Here's how the part is built. I have some questions about the finished solid (model axes, mm). A direction names the side the tool comes from. Coordinates: 2 decimals unless noted, no trailing zeros. Write each loop counter-clockwise with the first axis right and the second up, starting at its lowest first coordinate (ties: lowest second). Pieces come first, ordered by that corner, then holes.
Item 1: I want a section at B-B (z = -5). Please give me the cut outline in (x, y) (3 decimals), and give its area (3 significant figures).
Item 2: I want a section at C-C (y = 10.25). Please give me the cut outline in (x, z) (3 decimals).
Item 3: Please list where these lines run through material, in increasing order: line 1 (Y direction, x = 25, z = 0.5); line 2 (X direction, y = 3, z = 0.75) (3 decimals); line 3 (X direction, y = 4.5, z = -3) (3 decimals).
Item 4: If we mould it in two halves opening along X, with no side actions, what happens to faces 4 (the face through (62.103, 10, 3)), 5 (the face through (61.595, 10, 3)), 6 (the face through (22.71, 21.45, 0.09))? For each: pulls with the +X half, pulls with the -X half, needs draft (parallel to the pull), parting line crosses it, or undercut.
Item 5: I want a section at A-A (x = 52.5). Please give me the cut outline in (y, z), and give its area (3 significant figures).
Item 6: I want a section at D-D (z = 2.75). Please give me the cut outline in (x, y) (3 decimals), and give its area (3 significant figures).
Item 7: For faces 1 (the face through (1, 0.508, 0)), 2 (the face through (61.213, 20.72, 0.088)), 3 (the face through (1, 0, 0)), which set-ups out of +Z, -Z, +X, -X, +Y, -Y let a thin tool reach every point of the face, with its end or its side?
Item 8: I'm going to push flat-ended pins straight in: P1, Ø4, axis at x = 45.5, z = -1.5, coming from the +Y side; P2, Ø4, axis at x = 45, z = 0, coming from the -Y side; P3, Ø4, axis at y = 12.5, z = -4, coming from the -X side; P4, Ø0.6, axis at x = 62, z = -1, coming from the +Y side. Where does each tip first touch, or does it pass through?
from build123d import *

# Parameters (mm, degrees)
EXTRUDE_THIN1_DEPTH = 6.3119
CUT_EXTRUDE1_REACH  = 68.051
SKETCH2_W           = 4.318
SKETCH2_H           = 11.049
CUT_EXTRUDE2_REACH  = 68.051
SKETCH3_R           = 1.524
SKETCH3_R_2         = 3.4925


with BuildPart() as part:
    # Sketch1 → Extrude-Thin1 (new, symmetric)
    with BuildSketch(Plane.XY):
        with BuildLine():
            Line((0, 0), (1.784287341, 0))
            ThreePointArc((1.784287341, 0), (2.479784243, 0.141672386), (3.064445706, 0.54411242))
            Line((3.064445706, 0.54411242), (22.485395925, 20.693348272))
            ThreePointArc((22.485395925, 20.693348272), (22.903011255, 20.980805438), (23.399794757, 21.082))
            Line((23.399794757, 21.082), (60.325, 21.082))
            ThreePointArc((60.325, 21.082), (61.223025612, 20.710025612), (61.595, 19.812))
            Line((61.595, 19.812), (61.595, 0))
            Line((61.595, 0), (62.103, 0))
            Line((62.103, 0), (62.103, 19.812))
            ThreePointArc((62.103, 19.812), (61.582235857, 21.069235857), (60.325, 21.59))
            Line((60.325, 21.59), (23.399794757, 21.59))
            ThreePointArc((23.399794757, 21.59), (22.704297854, 21.448327614), (22.119636392, 21.04588758))
            Line((22.119636392, 21.04588758), (2.698686173, 0.896651728))
            ThreePointArc((2.698686173, 0.896651728), (2.281070842, 0.609194562), (1.784287341, 0.508))
            Line((1.784287341, 0.508), (0, 0.508))
            Line((0, 0.508), (0, 0))
        make_face()
    extrude(amount=EXTRUDE_THIN1_DEPTH, both=True)

    # Sketch2 → Cut-Extrude1 (cut, up to next)
    with BuildSketch(Plane(origin=(62.103, 0, 0), x_dir=(0, 0, -1), z_dir=(1, 0, 0)), mode=Mode.PRIVATE) as cut_extrude1_sk1:
        with Locations((0, 11.4935)):
            Rectangle(SKETCH2_W, SKETCH2_H)
    cut_extrude1_tool1 = extrude(cut_extrude1_sk1.sketch, amount=-CUT_EXTRUDE1_REACH, mode=Mode.PRIVATE) & part.part
    add(cut_extrude1_tool1.solids().sort_by_distance((62.103, 11.4935, 0))[0], mode=Mode.SUBTRACT)

    # Sketch3 → Cut-Extrude2 (cut, up to next)
    with BuildSketch(Plane(origin=(0, 21.59, 0), x_dir=(1, 0, 0), z_dir=(0, 1, 0)), mode=Mode.PRIVATE) as cut_extrude2_sk1:
        with Locations(Location((52.7812, 0, 0), (0, 0, 180))):
            Circle(SKETCH3_R)
    cut_extrude2_tool1 = extrude(cut_extrude2_sk1.sketch, amount=-CUT_EXTRUDE2_REACH, mode=Mode.PRIVATE) & part.part
    # Sketch3 → Cut-Extrude2 (cut, up to next)
    with BuildSketch(Plane(origin=(0, 21.59, 0), x_dir=(1, 0, 0), z_dir=(0, 1, 0)), mode=Mode.PRIVATE) as cut_extrude2_sk2:
        with Locations(Location((32.8422, 0, 0), (0, 0, 180))):
            Circle(SKETCH3_R)
    cut_extrude2_tool2 = extrude(cut_extrude2_sk2.sketch, amount=-CUT_EXTRUDE2_REACH, mode=Mode.PRIVATE) & part.part
    # Sketch3 → Cut-Extrude2 (cut, up to next)
    with BuildSketch(Plane(origin=(0, 21.59, 0), x_dir=(1, 0, 0), z_dir=(0, 1, 0)), mode=Mode.PRIVATE) as cut_extrude2_sk3:
        with Locations(Location((43.9547, 0, 0), (0, 0, 180))):
            Circle(SKETCH3_R_2)
    cut_extrude2_tool3 = extrude(cut_extrude2_sk3.sketch, amount=-CUT_EXTRUDE2_REACH, mode=Mode.PRIVATE) & part.part
    add(cut_extrude2_tool1.solids().sort_by_distance((52.7812, 21.59, 0))[0], mode=Mode.SUBTRACT)
    add(cut_extrude2_tool2.solids().sort_by_distance((32.8422, 21.59, 0))[0], mode=Mode.SUBTRACT)
    add(cut_extrude2_tool3.solids().sort_by_distance((43.9547, 21.59, 0))[0], mode=Mode.SUBTRACT)


solid = part.part
Answer:
1. outline: (0, 0) - (1.784, 0) arc R1.778 ccw to (3.064, 0.544) - (22.485, 20.693) arc R1.27 cw to (23.4, 21.082) - (60.325, 21.082) arc R1.27 cw to (61.595, 19.812) - (61.595, 0) - (62.103, 0) - (62.103, 19.812) arc R1.778 ccw to (60.325, 21.59) - (23.4, 21.59) arc R1.778 ccw to (22.12, 21.046) - (2.699, 0.897) arc R1.27 cw to (1.784, 0.508) - (0, 0.508) - close
1. area: 46.4 mm2
2. outline: (11.714, -6.312) - (12.42, -6.312) - (12.42, 6.312) - (11.714, 6.312) - close; (61.595, -6.312) - (62.103, -6.312) - (62.103, -2.159) - (61.595, -2.159) - close; (61.595, 2.159) - (62.103, 2.159) - (62.103, 6.312) - (61.595, 6.312) - close
3. line 1: y = 21.08 to 21.59
3. line 2: x = 4.726 to 5.432, 61.595 to 62.103
3. line 3: x = 6.172 to 6.877, 61.595 to 62.103
4. face 4: pulls with the +X half
4. face 5: undercut
4. face 6: pulls with the -X half
5. outline: (21.08, -6.31) - (21.59, -6.31) - (21.59, -1.5) - (21.08, -1.5) - close; (21.08, 1.5) - (21.59, 1.5) - (21.59, 6.31) - (21.08, 6.31) - close
5. area: 4.89 mm2
6. outline: (0, 0) - (1.784, 0) arc R1.778 ccw to (3.064, 0.544) - (22.485, 20.693) arc R1.27 cw to (23.4, 21.082) - (41.802, 21.082) - (41.802, 21.59) - (23.4, 21.59) arc R1.778 ccw to (22.12, 21.046) - (2.699, 0.897) arc R1.27 cw to (1.784, 0.508) - (0, 0.508) - close; (46.108, 21.082) - (60.325, 21.082) arc R1.27 cw to (61.595, 19.812) - (61.595, 0) - (62.103, 0) - (62.103, 19.812) arc R1.778 ccw to (60.325, 21.59) - (46.108, 21.59) - close
6. area: 44.2 mm2
7. face 1: +Z, -Z, -X, +Y
7. face 2: +Z, -Z, -Y
7. face 3: +Z, -Z, +X, -X, -Y
8. P1: stops at y = 21.59
8. P2: passes through
8. P3: stops at x = 11.95
8. P4: stops at y = 20.94
